Check sheet for the modelled part. Datum: model origin and axes. Units: mm. A direction names the side the tool comes from. Coordinates: 2 decimals unless noted, no trailing zeros. Order: outer loops, then holes, each group sorted by start corner. A loop starts at its lowest first (then second) coordinate and runs counter-clockwise, first axis right, second up.
1. Cross-section at B-B (z = -22). Enter the section's corners in (x, y).
2. Cross-section at C-C (y = -5). Enter the section's corners in (x, z), then the cut area to 3 significant figures.
3. Set-up check for faces 4 (the flat face through (0, -22.5, -57)), 5 (the cylindrical face through (0.089, -12.444, 27.406)): record each of +Z, -Z, +X, -X, +Y, -Y from which the full face is reachable in a straight line by a thin tool's end or side.
4. Draft check along Y on faces 1 (the cylindrical face through (-1.846, -86.73, 40.095)), 2 (the flat face through (0, 0, -100)), 3 (the cylindrical face through (-0.09, -98.96, 22.26)). Enter one of: released by +Y, released by -Y, zero draft, split by the parting line, or undercut.
5. Cross-section at A-A (y = 17.5). Enter the section's corners in (x, z).
6. Thickness scan on line 1 (Y direction, x = 2.5, z = -35); line 2 (X direction, y = 5, z = -92); line 3 (Y direction, x = 1.75, z = 21). Record the ranges inside material, lowest first.
7. Gauge pin test, flat ends, axial feed: pin 1 Ø1.5 at (x, y) = (2, -32) entering from +Z; pin 2 Ø4 at (x, y) = (2, -77.5) entering from +Z; pin 3 Ø6.5 at (x, z) = (-2.5, -37.5) entering from -Y. Record the tip position at first contact, or that the pin passes through.
8. Cross-section at D-D (x = 1.25). Count the separate pieces of the cut face and the enclosed holes in it, then the cut area to 3 significant figures.
```python
from build123d import *

# Parameters (mm, degrees)
CROQUIS1_R                    = 9
SALIENTE_EXTRUIR1_DEPTH       = 6.35
DI_METRO_DE_TALADRO_5_0_5_1_D = 8
DI_METRO_DE_TALADRO_5_0_5_2_D = 8
REDONDEO1_R                   = 3
TALADRO_ROSCADO_M4X0_71_D     = 3.3
TALADRO_DE_MARGEN_PARA_M41_D  = 4.5


with BuildPart() as part:
    # Croquis1 → Saliente-Extruir1 (new, symmetric)
    with BuildSketch(Plane(origin=(0, 0, 0), x_dir=(0, 0, -1), z_dir=(1, 0, 0))):
        Polygon((14.334080868, -22.5), (-21.869900966, -100.139689593), (-62.653751382, -81.121867814), (-14.334080868, 22.5), (100, 22.5), (100, -22.5), align=None)
        Circle(CROQUIS1_R, mode=Mode.SUBTRACT)
    extrude(amount=SALIENTE_EXTRUIR1_DEPTH, both=True)

    # Diámetro de taladro Ø5.0 (5)1 (through all)
    with Locations(Plane(origin=(0, 22.5, 0), x_dir=(1, 0, 0), z_dir=(0, 1, 0))):
        with Locations((0, 92), (0, 42)):
            Hole(DI_METRO_DE_TALADRO_5_0_5_1_D / 2)

    # Diámetro de taladro Ø5.0 (5)2 (through all)
    with Locations(Plane(origin=(0, 9.508910889, 20.391925208), x_dir=(1, 0, 0), z_dir=(0, 0.4226182617407033, 0.9063077870366483))):
        with Locations((0, -42), (0, -92)):
            Hole(DI_METRO_DE_TALADRO_5_0_5_2_D / 2)

    # Redondeo1
    redondeo1_edges = [part.edges().sort_by_distance(p)[0] for p in [
        (0, -22.5, -14.334080868),
        (0, -100.139689593, 21.869900966),
        (0, -81.121867814, 62.653751382),
        (0, 22.5, 14.334080868),
        (0, 22.5, -100),
        (0, -22.5, -100),
    ]]
    fillet(redondeo1_edges, radius=REDONDEO1_R)

    # Taladro roscado M4x0.71 (through all)
    with Locations(Plane.ZY.offset(6.35)):
        with Locations((10, 10), (-10, 10), (-10, -10), (10, -10)):
            Hole(TALADRO_ROSCADO_M4X0_71_D / 2)

    # Taladro de margen para M41 (through all)
    with Locations(Plane.ZY.offset(6.35)):
        with Locations((-6.562784515, -27.334590895), (-1.491365374, -38.21028434), (25.157988031, -12.542951734), (30.229407172, -23.418645179), (-22, 17.5), (-22, -17.5), (-34, 17.5), (-34, -17.5)):
            Hole(TALADRO_DE_MARGEN_PARA_M41_D / 2)


solid = part.part
```
Data:
1. outline: (-6.35, -22.5) - (6.35, -22.5) - (6.35, -19.75) - (-6.35, -19.75) - close; (-6.35, -15.25) - (6.35, -15.25) - (6.35, 15.25) - (-6.35, 15.25) - close; (-6.35, 19.75) - (6.35, 19.75) - (6.35, 22.5) - (-6.35, 22.5) - close
2. outline: (-6.35, -100) - (6.35, -100) - (6.35, -7.48) - (-6.35, -7.48) - close; (-6.35, 7.48) - (6.35, 7.48) - (6.35, 27.16) - (-6.35, 27.16) - close; hole circle Ø8 at (0, -92); hole circle Ø8 at (0, -42)
2. area: 1,320 mm2
3. face 4: -Z, +X, -X, -Y
3. face 5: +X, -X
4. face 1: undercut
4. face 2: zero draft
4. face 3: released by -Y
5. outline: (-6.35, -100) - (6.35, -100) - (6.35, -36.25) - (-6.35, -36.25) - close; (-6.35, -31.75) - (6.35, -31.75) - (6.35, -24.25) - (-6.35, -24.25) - close; (-6.35, -19.75) - (6.35, -19.75) - (6.35, 16.67) - (-6.35, 16.67) - close; hole circle Ø8 at (0, -92); hole circle Ø8 at (0, -42)
6. line 1: y = -22.5 to -19.52, -15.48 to 15.48, 19.52 to 22.5
6. line 2: x = -6.35 to -4, 4 to 6.35
6. line 3: y = -98.05 to -95.69, -87.75 to -40.52, -32.58 to 8.2
7. pin 1: stops at z = 40.1
7. pin 2: stops at z = 61.66
7. pin 3: stops at y = -22.5
8. separate pieces: 5
8. enclosed holes: 13
8. area: 7,210 mm2
